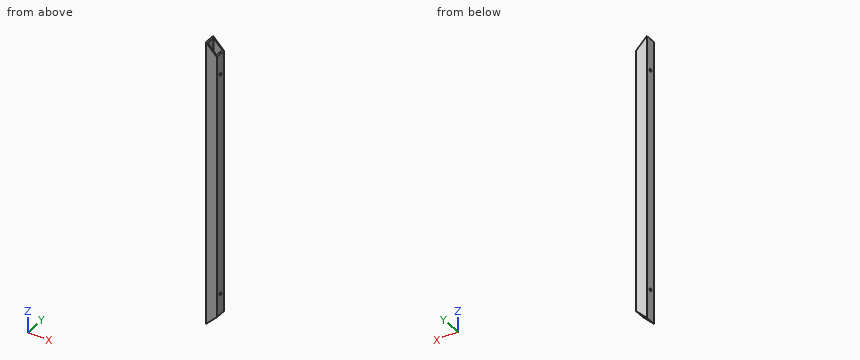
```python
from build123d import *

# Parameters (mm, degrees)
SKETCH1_W           = 50.8
SKETCH1_H           = 50.8
SKETCH1_W_2         = 41.275
SKETCH1_H_2         = 41.275
EXTRUDE_THIN1_DEPTH = 660.4
CUT_EXTRUDE1_DEPTH  = 51.8
SKETCH4_R           = 6.35
CUT_EXTRUDE2_DEPTH  = 51.8


with BuildPart() as part:
    # Sketch1 → Extrude-Thin1 (new body, symmetric)
    with BuildSketch(Plane.XY):
        with Locations((-254, 958.85)):
            Rectangle(SKETCH1_W, SKETCH1_H)
        with Locations((-254, 958.85)):
            Rectangle(SKETCH1_W_2, SKETCH1_H_2, mode=Mode.SUBTRACT)
    extrude(amount=EXTRUDE_THIN1_DEPTH, both=True)

    # Sketch3 → Cut-Extrude1 (cut, through all)
    with BuildSketch(Plane.XZ.offset(-933.45)):
        Polygon((-279.4, 660.4), (-228.6, 609.6), (-228.6, 660.4), align=None)
        Polygon((-279.4, -660.4), (-228.6, -609.6), (-228.6, -660.4), align=None)
    extrude(amount=-CUT_EXTRUDE1_DEPTH, mode=Mode.SUBTRACT)

    # Sketch4 → Cut-Extrude2 (cut, through all)
    with BuildSketch(Plane.ZY.offset(279.4)):
        with Locations((514.35, 958.85)):
            Circle(SKETCH4_R)
        with Locations((-514.35, 958.85)):
            Circle(SKETCH4_R)
    extrude(amount=-CUT_EXTRUDE2_DEPTH, mode=Mode.SUBTRACT)


solid = part.part
```
Build history of the part. All positions in model axes, mm. Give positions to 0.01 mm unless a question says otherwise; leave off trailing zeros. Loops run counter-clockwise (first coordinate to the right, second up) from the corner with the lowest first, then second, coordinate; pieces in that order, holes last. Notation, with made-up numbers: (74, 5) -> (106, 5) arc R31 ccw to (106, 40) -> close; hole circle Ø5 at (-15.5, 55). An arc over 180 degrees is marked (long way). One line per question, with ' | ' between items. Start each with the question number.
1) Probe L1, parallel to Y at x = -261.5, z = 166.5; L2, parallel to X at y = 950, z = -149.5; L3, parallel to Z at x = -277, y = 958.85. List the from-to ranges inside material, lowest first.
2) Cut at B-B (z = 238.5). Give the cut face in (x, y).
3) Pin check, flat tips, straight feed: pin 1 (4 mm diameter, centred on x = -235, y = 968, fed in from +Z); pin 2 (10 mm diameter, centred on x = -263, y = 942, fed in from -Z). Stop position of each tip, or through.
4) Cut at A-A (x = -242). Give the cut face in (y, z), plus the area to 3 significant figures.
Return value:
1) L1: 933.45 to 938.21, 979.49 to 984.25 | L2: -279.4 to -274.64, -233.36 to -228.6 | L3: -658 to -520.7, -508 to 508, 520.7 to 658
2) outline: (-279.4, 933.45) -> (-228.6, 933.45) -> (-228.6, 984.25) -> (-279.4, 984.25) -> close; hole (-274.64, 938.21) -> (-233.36, 938.21) -> (-233.36, 979.49) -> (-274.64, 979.49) -> close
3) pin 1: z = 614.36 | pin 2: z = -647.26
4) outline: (933.45, -623) -> (938.21, -623) -> (938.21, 623) -> (933.45, 623) -> close; (979.49, -623) -> (984.25, -623) -> (984.25, 623) -> (979.49, 623) -> close | area: 11,900 mm^2
